from build123d import *

# Parameters (mm, degrees)
F0_W     = 269.875
F0_H     = 76.2
F1_DEPTH = 38.1
F2_W     = 76.2
F2_H     = 914.4
F3_DEPTH = 38.1


with BuildPart() as f1:
    # F0 (on Top) → F1 (new body)
    with BuildSketch(Plane.XY):
        with Locations((134.9375, 38.1)):
            Rectangle(F0_W, F0_H)
    extrude(amount=F1_DEPTH)

    # F2 (on face) → F3 (join)
    with BuildSketch(Plane.YZ.offset(269.875)):
        with Locations((38.1, 457.2)):
            Rectangle(F2_W, F2_H)
    extrude(amount=F3_DEPTH)

    # F4: F1 across plane


with BuildPart() as f1_1:
    add(f1.part)
    add(f1.part.mirror(Plane.YZ))


solid = f1_1.part
Geometry check sheet. Reference: the model listing, model coordinates, mm. A direction names the side the tool comes from. Give positions to 0.01 mm unless a question says otherwise; leave off trailing zeros. Order: outer loops, then holes, each group sorted by start corner. A loop starts at its lowest first (then second) coordinate and runs counter-clockwise, first axis right, second up.
1) Draft check along X on faces 1 (the flat face through (4, 39, 38.1)), 2 (the flat face through (-289, 38, 914.4)), 3 (the flat face through (-269.875, 38, 482)), 4 (the flat face through (307.975, 38, 464)). Enter one of: released by +X, released by -X, zero draft, split by the parting line, or undercut.
Results are:
face 1: undercut
face 2: zero draft
face 3: undercut
face 4: released by +X
2) Cross-section at C-C (x = -232). Record the boundary of the cut face in (y, z).
Results are:
outline: (0, 0) - (76.2, 0) - (76.2, 38.1) - (0, 38.1) - close
3) Cross-section at B-B (y = 12). Record the boundary of the cut face in (x, z) (3 decimals), then the cut area to 3 significant figures.
Results are:
outline: (-307.975, 0) - (307.975, 0) - (307.975, 914.4) - (269.875, 914.4) - (269.875, 38.1) - (-269.875, 38.1) - (-269.875, 914.4) - (-307.975, 914.4) - close
area: 90,200 mm2
4) Material ranges on probe 1 along X at (y, z) = (45, 846.5) (3 decimals); probe 2 along Z at (x, y) = (-185, 38), recorded low to high.
Results are:
probe 1: x = -307.975 to -269.875, 269.875 to 307.975
probe 2: z = 0 to 38.1
5) Cross-section at A-A (z = 833). Record the boundary of the cut face in (x, y) (3 decimals).
Results are:
outline: (-307.975, 0) - (-269.875, 0) - (-269.875, 76.2) - (-307.975, 76.2) - close; (269.875, 0) - (307.975, 0) - (307.975, 76.2) - (269.875, 76.2) - close
6) Tool access check on faces 5 (the flat face through (269.875, 38, 482)), 6 (the flat face through (-307.975, 38, 464)). Record the directions out of +Z, -Z, +X, -X, +Y, -Y that give a thin tool (end or side, any length) a straight path to the whole face; none if there is none.
Results are:
face 5: +Z, +Y, -Y
face 6: +Z, -Z, -X, +Y, -Y
7) Gauge pin test, flat end, axial feed: pin 1 (3 mm diameter, centred on x = 183, y = 17.5, fed in from +Z). Record the tip position at first contact, or that the pin passes through.
Results are:
pin 1: stops at z = 38.1
